Part model, mm, in its own coordinate system. A direction names the side the tool comes from. Give positions to 0.01 mm unless a question says otherwise; leave off trailing zeros. Order: outer loops, then holes, each group sorted by start corner. A loop starts at its lowest first (then second) coordinate and runs counter-clockwise, first axis right, second up.
1. Mould opens along Z. For faces 3 (the cylindrical face through (1.5, 1.5, 0.6)), 4 (the flat face through (3, 1, 1)), 5 (the flat face through (1, 0, 2)), 6 (the cylindrical face through (2.4, 0, 0.6)) say: +Z half, -Z half, draft (parallel to the pull), parting line (faces both ways), or undercut.
2. Slice it at A-A on z = 4. List the corners of the cut face in (x, y).
3. Probe line 1 (Z direction, x = 1.5, y = 1.45); line 2 (Z direction, x = 1.5, y = 1.1); line 3 (X direction, y = 1.75, z = 4). List the from-to ranges inside material, lowest first.
4. Which spindle directions (+Z, -Z, +X, -X, +Y, -Y) get a long thin tool onto all of the face, cutting with end or side? Do faces 1 (the flat face through (2.2, 1.2, 4.5)), 2 (the cylindrical face through (1.5, 1.9, 4.6)). Say none if no direction does.
5. Slice it at B-B on x = 2.2. List the corners of the cut face in (y, z), and give its area (3 significant figures).
6. Slice it at C-C on y = -0.1. List the corners of the cut face in (x, z), and give its area (3 significant figures).
7. Drop flat-ended pins along their axis: pin 1 Ø1.4 at (x, z) = (1.5, 4) entering from -Y; pin 2 Ø1.4 at (x, y) = (1.5, -1) entering from +Z. Give the stop position or say it passes through.
8. Slice it at D-D on z = 0.5. List the corners of the cut face in (x, y), and give its area (3 significant figures).
from build123d import *

# Parameters (mm, degrees)
SKETCH_1_W               = 4
SKETCH_1_H               = 2.5
SKETCH_1_R               = 0.6
SKETCH_1_H_2             = 1.5
EXTRUDE_1_DEPTH          = 3
CUT_EXTRUDE_1_DEPTH      = 8.158910532
CUT_EXTRUDE_1_DEPTH_BACK = 8.158910532
SKETCH_3_R               = 0.6
SKETCH_5_W               = 4
SKETCH_5_H               = 0.2
CUT_EXTRUDE_2_DEPTH      = 8.158910532


with BuildPart() as part:
    # 草图1 → 凸台-拉伸1 (new body)
    # profile 1 of 3: a face of its own
    with BuildSketch(Plane(origin=(0, 0, 0), x_dir=(0, 0, -1), z_dir=(1, 0, 0))):
        with Locations((0, -0.25)):
            Rectangle(SKETCH_1_W, SKETCH_1_H)
        Circle(SKETCH_1_R, mode=Mode.SUBTRACT)
    # profile 2 of 3: a face of its own
    with BuildSketch(Plane(origin=(0, 0, 0), x_dir=(0, 0, -1), z_dir=(1, 0, 0))):
        with Locations((0, 1.75)):
            Rectangle(SKETCH_1_W, SKETCH_1_H_2)
    # profile 3 of 3: a face of its own
    with BuildSketch(Plane(origin=(0, 0, 0), x_dir=(0, 0, -1), z_dir=(1, 0, 0))):
        with Locations((-4, 1.75)):
            Rectangle(SKETCH_1_W, SKETCH_1_H_2)
    extrude(amount=EXTRUDE_1_DEPTH)

    # 草图3 → 切除-拉伸1 (cut, two sides: drawn at the far end of the back side and taken through both)
    with BuildSketch(Plane.XZ.offset(-1).offset(-CUT_EXTRUDE_1_DEPTH_BACK)):
        with Locations(Location((1.5, 4, 0), (0, 0, 270))):
            Circle(SKETCH_3_R)
        with Locations(Location((1.5, 0, 0), (0, 0, 270))):
            Circle(SKETCH_3_R)
    extrude(amount=CUT_EXTRUDE_1_DEPTH + CUT_EXTRUDE_1_DEPTH_BACK, mode=Mode.SUBTRACT)

    # 草图5 → 切除-拉伸2 (cut, through all)
    with BuildSketch(Plane(origin=(3, 0, 0), x_dir=(0, 0, -1), z_dir=(1, 0, 0))):
        with Locations((-4, 1.1)):
            Rectangle(SKETCH_5_W, SKETCH_5_H)
    extrude(amount=-CUT_EXTRUDE_2_DEPTH, mode=Mode.SUBTRACT)


solid = part.part
Data:
1. face 3: undercut
1. face 4: draft
1. face 5: +Z half
1. face 6: undercut
2. outline: (0, 1.2) - (0.9, 1.2) - (0.9, 2.5) - (0, 2.5) - close; (2.1, 1.2) - (3, 1.2) - (3, 2.5) - (2.1, 2.5) - close
3. line 1: z = -2 to -0.6, 0.6 to 3.4, 4.6 to 6
3. line 2: z = -2 to -0.6, 0.6 to 2
3. line 3: x = 0 to 0.9, 2.1 to 3
4. face 1: +Z, +X, -X, -Y
4. face 2: +Y, -Y
5. outline: (-1.5, -2) - (2.5, -2) - (2.5, 6) - (1.2, 6) - (1.2, 2) - (-1.5, 2) - close; hole circle Ø1.2 at (0, 0)
5. area: 20.1 mm2
6. outline: (0, -2) - (3, -2) - (3, -0.59) - (1.6, -0.59) arc R0.6 cw to (1.4, -0.59) - (0, -0.59) - close; (0, 0.59) - (1.4, 0.59) arc R0.6 cw to (1.6, 0.59) - (3, 0.59) - (3, 2) - (0, 2) - close
6. area: 8.45 mm2
7. pin 1: stops at y = 1.2
7. pin 2: stops at z = 2
8. outline: (0, -1.5) - (1.17, -1.5) - (1.17, -0.33) - (0, -0.33) - close; (0, 0.33) - (1.17, 0.33) - (1.17, 2.5) - (0, 2.5) - close; (1.83, -1.5) - (3, -1.5) - (3, -0.33) - (1.83, -0.33) - close; (1.83, 0.33) - (3, 0.33) - (3, 2.5) - (1.83, 2.5) - close
8. area: 7.80 mm2
